Job drawing, mm, ordinate dimensions from the low corner. One solid piece. Give positions to 0.01 mm unless a question says otherwise; leave off trailing zeros. Write each loop counter-clockwise with the first axis right and the second up, starting at its lowest first coordinate (ties: lowest second). Pieces come first, ordered by that corner, then holes. Notation, with made-up numbers: M -33,10.25 L 24,10.25 A21 cw 24,42.25 Z; hole C 8,88.25 d6. An arc over 180 degrees is marked long. Use a Markdown table: item, result.
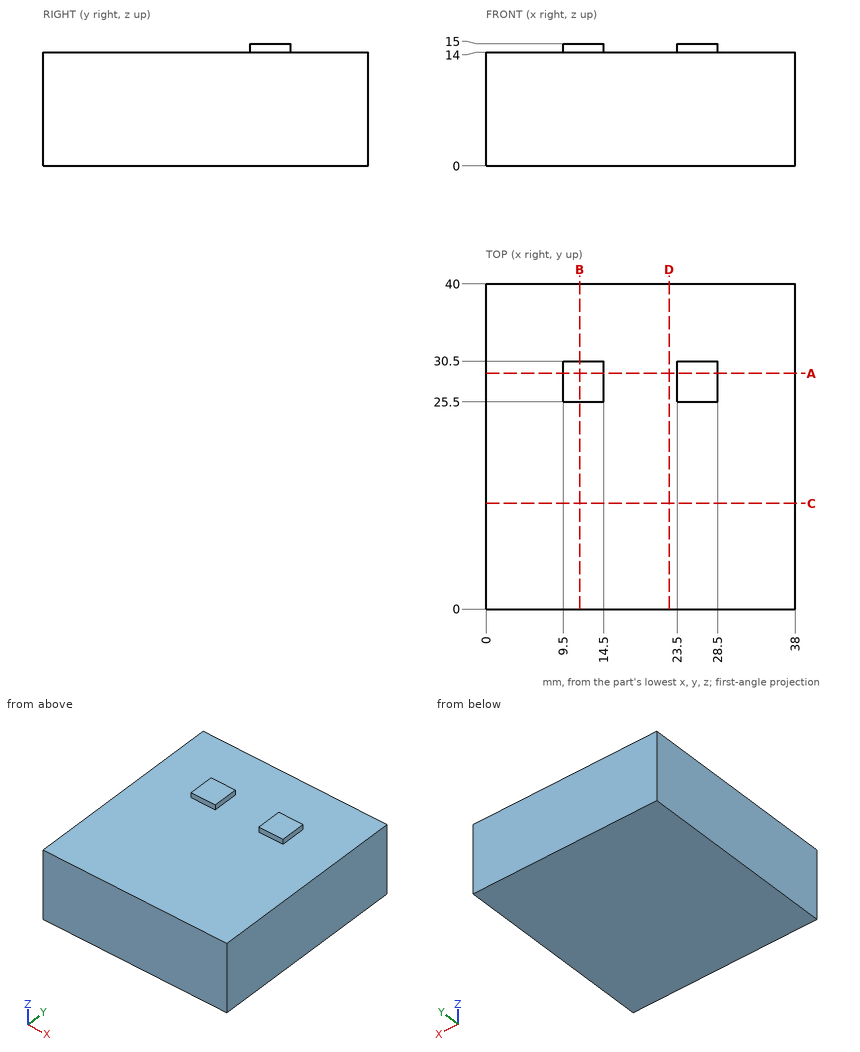
1. Drop flat-ended pins along their axis: P1, Ø0.5, axis at y = 27.5, z = 14.5, coming from the +X side; P2, Ø19, axis at x = 24.5, y = 18.5, coming from the +Z side; P3, Ø0.8, axis at x = 25.5, z = 14.5, coming from the +Y side; P4, Ø0.5, axis at y = 29, z = 14.5, coming from the -X side. Give the stop position or say it passes through.
Findings below:
| item | result |
|---|---|
| P1 | x = 28.5 |
| P2 | z = 15 |
| P3 | y = 30.5 |
| P4 | x = 9.5 |
2. Cut at D-D, the plane x = 22.5. Give the cut face in (y, z), then the cut area to 3 significant figures.
Findings below:
| item | result |
|---|---|
| outline | M 0,0 L 40,0 L 40,14 L 0,14 Z |
| area | 560 mm2 |
3. Cut at C-C, the plane y = 13. Give the cut face in (x, z).
Findings below:
| item | result |
|---|---|
| outline | M 0,0 L 38,0 L 38,14 L 0,14 Z |
4. Drill centre line: L1, parallel to Z at x = 25, y = 10. Where is it in solid material? Low to high.
Findings below:
| item | result |
|---|---|
| L1 | 0 to 14 |
5. Cut at B-B, the plane x = 11.5. Give the cut face in (y, z), then the cut area to 3 significant figures.
Findings below:
| item | result |
|---|---|
| outline | M 0,0 L 40,0 L 40,14 L 30.5,14 L 30.5,15 L 25.5,15 L 25.5,14 L 0,14 Z |
| area | 565 mm2 |
6. Cut at A-A, the plane y = 29. Give the cut face in (x, z).
Findings below:
| item | result |
|---|---|
| outline | M 0,0 L 38,0 L 38,14 L 28.5,14 L 28.5,15 L 23.5,15 L 23.5,14 L 14.5,14 L 14.5,15 L 9.5,15 L 9.5,14 L 0,14 Z |
